```python
from build123d import *

# Parameters (mm, degrees)
F0_W      = 152.4
F0_H      = 75.6477481976
F1_DEPTH  = 25.4
F2_W      = 50.8
F2_H      = 25.4
F3_DEPTH  = 381
F4_W      = 25.4
F4_H      = 12.7
F5_DEPTH  = 63.5
F6_W      = 25.4
F6_H      = 12.7
F7_DEPTH  = 63.5
F8_W      = 25.4
F8_H      = 12.7
F9_DEPTH  = 63.5
F10_W     = 25.4
F10_H     = 12.7
F11_DEPTH = 63.5
F12_W     = 25.4
F12_H     = 12.7
F13_DEPTH = 25.4
F14_W     = 25.4
F14_H     = 12.7
F18_DEPTH = 25.4
F15_W     = 24.92688122
F15_H     = 12.7
F19_DEPTH = 25.4
F16_W     = 24.9687274059
F16_H     = 12.7
F20_DEPTH = 25.4
F17_W     = 25.0190113743
F17_H     = 12.7
F21_DEPTH = 25.4
F22_W     = 25.4
F22_H     = 12.7
F27_DEPTH = 25.4
F23_W     = 25.320323884
F23_H     = 12.7
F28_DEPTH = 25.4
F24_W     = 25.3337946793
F24_H     = 12.7
F29_DEPTH = 25.4
F25_W     = 25.1309572571
F25_H     = 12.7
F30_DEPTH = 25.4
F26_W     = 25.4
F26_H     = 12.7
F31_DEPTH = 25.4


with BuildPart() as f1:
    # F0 (on Top) → F1 (new body)
    with BuildSketch(Plane.XY):
        with Locations((-1.49496e-05, -37.8238740988)):
            Rectangle(F0_W, F0_H)
    extrude(amount=F1_DEPTH)

    # F2 (on face) → F3 (join)
    with BuildSketch(Plane.XY.offset(25.4)):
        with Locations((-0.9335875511, -33.0558609421)):
            Rectangle(F2_W, F2_H)
    extrude(amount=F3_DEPTH)

    # F4 (on face) → F5 (join)
    with BuildSketch(Plane.YZ.offset(24.4664124489)):
        with Locations((-33.0558609421, 400.05)):
            Rectangle(F4_W, F4_H)
    extrude(amount=F5_DEPTH)

    # F6 (on face) → F7 (join)
    with BuildSketch(Plane.YZ.offset(24.4664124489)):
        with Locations((-33.0558609421, 369.57)):
            Rectangle(F6_W, F6_H)
    extrude(amount=F7_DEPTH)

    # F8 (on face) → F9 (join)
    with BuildSketch(Plane(origin=(-26.3335875511, 0, 0), x_dir=(0, -1, 0), z_dir=(-1, 0, 0))):
        with Locations((33.0558609421, 400.05)):
            Rectangle(F8_W, F8_H)
    extrude(amount=F9_DEPTH)

    # F10 (on face) → F11 (join)
    with BuildSketch(Plane(origin=(-26.3335875511, 0, 0), x_dir=(0, -1, 0), z_dir=(-1, 0, 0))):
        with Locations((33.0558609421, 369.57)):
            Rectangle(F10_W, F10_H)
    extrude(amount=F11_DEPTH)

    # F12 (on face) → F13 (join)
    with BuildSketch(Plane.YZ.offset(24.4664124489)):
        with Locations((-33.0558609421, 323.85)):
            Rectangle(F12_W, F12_H)
    extrude(amount=F13_DEPTH)

    # F14 (on face) → F18 (join)
    with BuildSketch(Plane.YZ.offset(24.4664124489)):
        with Locations((-33.0558609421, 286.004)):
            Rectangle(F14_W, F14_H)
    extrude(amount=F18_DEPTH)

    # F15 (on face) → F19 (join)
    with BuildSketch(Plane.YZ.offset(24.4664124489)):
        with Locations((-32.8193015521, 248.158)):
            Rectangle(F15_W, F15_H)
    extrude(amount=F19_DEPTH)

    # F16 (on face) → F20 (join)
    with BuildSketch(Plane.YZ.offset(24.4664124489)):
        with Locations((-32.840224645, 204.978)):
            Rectangle(F16_W, F16_H)
    extrude(amount=F20_DEPTH)

    # F17 (on face) → F21 (join)
    with BuildSketch(Plane.YZ.offset(24.4664124489)):
        with Locations((-32.8653666293, 161.798)):
            Rectangle(F17_W, F17_H)
    extrude(amount=F21_DEPTH)

    # F22 (on face) → F27 (join)
    with BuildSketch(Plane(origin=(-26.3335875511, 0, 0), x_dir=(0, -1, 0), z_dir=(-1, 0, 0))):
        with Locations((33.0558609421, 323.85)):
            Rectangle(F22_W, F22_H)
    extrude(amount=F27_DEPTH)

    # F23 (on face) → F28 (join)
    with BuildSketch(Plane(origin=(-26.3335875511, 0, 0), x_dir=(0, -1, 0), z_dir=(-1, 0, 0))):
        with Locations((33.0956990001, 286.004)):
            Rectangle(F23_W, F23_H)
    extrude(amount=F28_DEPTH)

    # F24 (on face) → F29 (join)
    with BuildSketch(Plane(origin=(-26.3335875511, 0, 0), x_dir=(0, -1, 0), z_dir=(-1, 0, 0))):
        with Locations((33.0227582817, 248.158)):
            Rectangle(F24_W, F24_H)
    extrude(amount=F29_DEPTH)

    # F25 (on face) → F30 (join)
    with BuildSketch(Plane(origin=(-26.3335875511, 0, 0), x_dir=(0, -1, 0), z_dir=(-1, 0, 0))):
        with Locations((32.9213395706, 204.978)):
            Rectangle(F25_W, F25_H)
    extrude(amount=F30_DEPTH)

    # F26 (on face) → F31 (join)
    with BuildSketch(Plane(origin=(-26.3335875511, 0, 0), x_dir=(0, -1, 0), z_dir=(-1, 0, 0))):
        with Locations((33.0558609421, 161.798)):
            Rectangle(F26_W, F26_H)
    extrude(amount=F31_DEPTH)


solid = f1.part
```
Geometry check sheet. Reference: the model listing, model coordinates, mm. A direction names the side the tool comes from. Give positions to 0.01 mm unless a question says otherwise; leave off trailing zeros. Write each loop counter-clockwise with the first axis right and the second up, starting at its lowest first coordinate (ties: lowest second). Pieces come first, ordered by that corner, then holes. Notation, with made-up numbers: (24, 43) - (31, 43) arc R23 cw to (31, 70) - close; hole circle Ø3 at (-37, 44.25). An arc over 180 degrees is marked (long way). Use a Markdown table: item, result.
Q1. Set-up check for faces 1 (the face through (-76.2, -38, 13)), 2 (the face through (37, -33, 292.354)), 3 (the face through (-26.334, -33, 346)): record each of +Z, -Z, +X, -X, +Y, -Y from which the full face is reachable in a straight line by a thin tool's end or side.
Computed:
| item | result |
|---|---|
| face 1 | -Z, -X, +Y, -Y |
| face 2 | +X, +Y, -Y |
| face 3 | -X, +Y, -Y |
Q2. Section check C-C, the plane z = 288.5. Enter the section's corners in (x, y).
Computed:
| item | result |
|---|---|
| outline | (-51.73, -45.76) - (49.87, -45.76) - (49.87, -20.36) - (-26.33, -20.36) - (-26.33, -20.44) - (-51.73, -20.44) - close |
Q3. Thickness scan on L1, parallel to Z at x = -64, y = -42; L2, parallel to Z at x = 45.5, y = -53; L3, parallel to X at y = -69, z = 25. Record the ranges inside material, lowest first. Write a range as [from, to].
Computed:
| item | result |
|---|---|
| L1 | z = [0, 25.4], [363.22, 375.92], [393.7, 406.4] |
| L2 | z = [0, 25.4] |
| L3 | x = [-76.2, 76.2] |
Q4. Section check A-A, the plane x = -36.5. Give the number of separate pieces and of enclosed holes in the cut face, then the cut area to 3 significant figures.
Computed:
| item | result |
|---|---|
| separate pieces | 8 |
| enclosed holes | 0 |
| area | 4,170 mm² |
Q5. Section check B-B, the plane x = 56. Enter the section's corners in (y, z).
Computed:
| item | result |
|---|---|
| outline | (-75.65, 0) - (0, 0) - (0, 25.4) - (-75.65, 25.4) - close; (-45.76, 363.22) - (-20.36, 363.22) - (-20.36, 375.92) - (-45.76, 375.92) - close; (-45.76, 393.7) - (-20.36, 393.7) - (-20.36, 406.4) - (-45.76, 406.4) - close |
Q6. Go/stop test with flat-tipped pins: P1, Ø5, axis at x = -4, z = 85.5, coming from the +Y side; P2, Ø5, axis at x = -60.5, y = -58, coming from the +Z side; P3, Ø6.5, axis at x = 33.5, z = 165, coming from the -Y side. Record where each tip stops, or that it passes through.
Computed:
| item | result |
|---|---|
| P1 | stops at y = -20.36 |
| P2 | stops at z = 25.4 |
| P3 | stops at y = -45.37 |
